Source: three-view drawing plus pictorial views. Frame: mm from the lowest corner of the part. Coordinates: 2 decimals unless noted, no trailing zeros. Order: outer loops, then holes, each group sorted by start corner. A loop starts at its lowest first (then second) coordinate and runs counter-clockwise, first axis right, second up. Notation, with made-up numbers: (65, -2) -> (72, -2) arc R16 cw to (72, 27) -> close; hole circle Ø9 at (86, 45). An arc over 180 degrees is marked (long way). One line per question, with ' | ' between items.
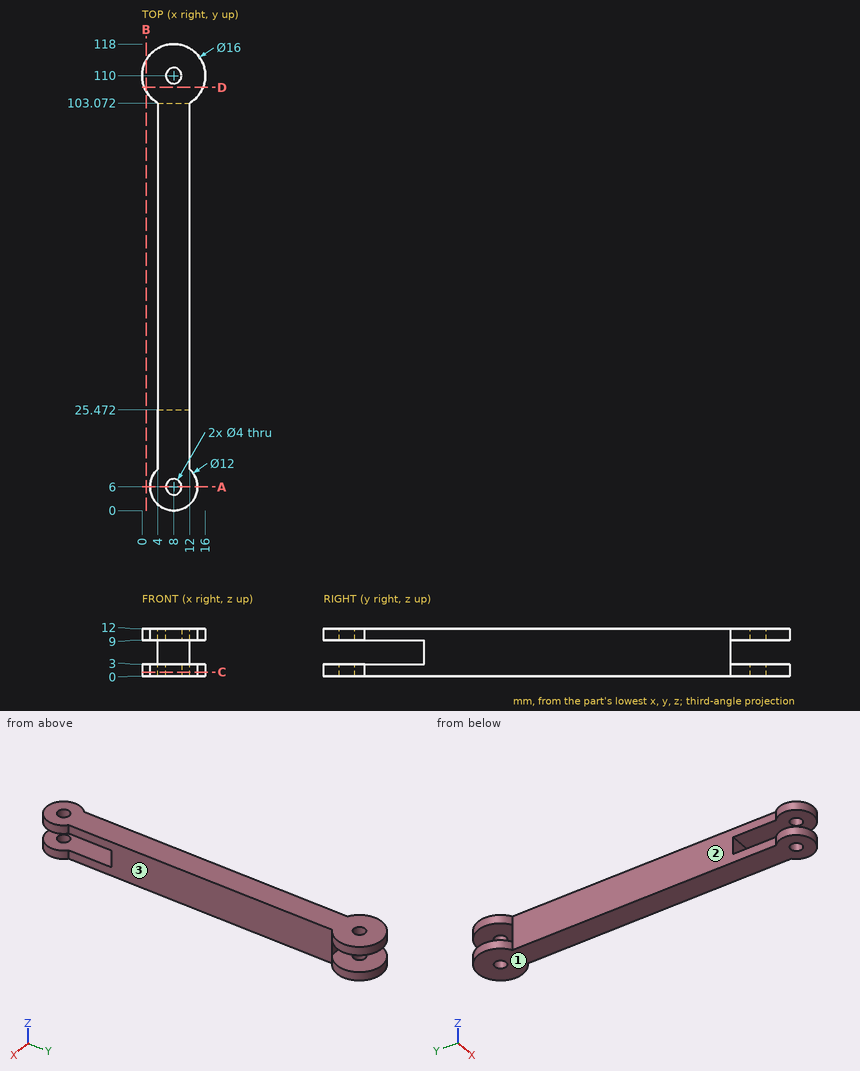
1. Cut plane B-B, the plane x = 1. Return loops of the section in (y, z), and give its area (3 significant figures).
Recorded:
outline: (106.13, 0) -> (113.87, 0) -> (113.87, 3) -> (106.13, 3) -> close; (106.13, 9) -> (113.87, 9) -> (113.87, 12) -> (106.13, 12) -> close | area: 46.5 mm^2
2. Cut plane C-C, the plane z = 1. Return loops of the section in (x, y).
Recorded:
outline: (4, 10.47) arc R6 ccw (long way) to (12, 10.47) -> (12, 103.07) arc R8 ccw (long way) to (4, 103.07) -> close; hole circle Ø4 at (8, 6); hole circle Ø4 at (8, 110)
3. Cut plane D-D, the plane y = 107. Return loops of the section in (x, z), and give its area (3 significant figures).
Recorded:
outline: (0.58, 0) -> (15.42, 0) -> (15.42, 3) -> (0.58, 3) -> close; (0.58, 9) -> (15.42, 9) -> (15.42, 12) -> (0.58, 12) -> close | area: 89.0 mm^2
4. Mould query, pull axis Y, two halves, no side actions, for the marked faces 1, 2 and 3. Classes: released by +Y, released by -Y, zero draft, split by the parting line, or undercut.
Recorded:
face 1: zero draft | face 2: undercut | face 3: undercut
5. Pin query (flat end, axial travel): pin 1 Ø6 at (y, z) = (45.5, 5) entering from -X; pin 2 Ø5 at (x, z) = (3, 7.5) entering from +Y; pin 3 Ø1.8 at (x, z) = (8, 6.5) entering from -Y. Return the tip coordinate at first contact, or that it passes through.
Recorded:
pin 1: stops at x = 4 | pin 2: stops at y = 117.42 | pin 3: stops at y = 25.47
6. Ray query, line 1 (Y direction, x = 8, z = 10.2); line 2 (X direction, y = 110, z = 10.85); line 3 (Z direction, x = 12.5, y = 5). Return the intervals inside material, ascending. Write a range as [from, to].
Recorded:
line 1: y = [0, 4], [8, 108], [112, 118] | line 2: x = [0, 6], [10, 16] | line 3: z = [0, 3], [9, 12]
7. Cut plane A-A, the plane y = 6. Return loops of the section in (x, z).
Recorded:
outline: (2, 0) -> (6, 0) -> (6, 3) -> (2, 3) -> close; (2, 9) -> (6, 9) -> (6, 12) -> (2, 12) -> close; (10, 0) -> (14, 0) -> (14, 3) -> (10, 3) -> close; (10, 9) -> (14, 9) -> (14, 12) -> (10, 12) -> close
